from build123d import *

# Parameters (mm, degrees)
SKETCH1_W                  = 174
SKETCH1_H                  = 18
BOSS_EXTRUDE1_DEPTH        = 46
SKETCH3_W                  = 126
SKETCH3_H                  = 46
CUT_EXTRUDE1_DEPTH         = 4
SKETCH4_R                  = 7
BOSS_EXTRUDE2_DEPTH        = 14
SKETCH5_R                  = 14
SKETCH5_R_2                = 7
BOSS_EXTRUDE3_DEPTH        = 2
RIB1_REACH                 = 162.545
SKETCH6_WALL_W             = 359.980893116
SKETCH6_WALL_H             = 10
FILLET1_R                  = 2
FILLET2_R                  = 2
FILLET3_R                  = 2
F_10_0_10_DIAMETER_HOLE5_D = 10


with BuildPart() as part:
    # Sketch1 → Boss-Extrude1 (new body)
    with BuildSketch(Plane.XY):
        with Locations((54.12605042, 9)):
            Rectangle(SKETCH1_W, SKETCH1_H)
    extrude(amount=-BOSS_EXTRUDE1_DEPTH)

    # Sketch3 → Cut-Extrude1 (cut)
    with BuildSketch(Plane(origin=(0, 18, 0), x_dir=(1, 0, 0), z_dir=(0, 1, 0))):
        with Locations((54.12605042, 23)):
            Rectangle(SKETCH3_W, SKETCH3_H)
    extrude(amount=-CUT_EXTRUDE1_DEPTH, mode=Mode.SUBTRACT)

    # Sketch4 → Boss-Extrude2 (add)
    with BuildSketch(Plane(origin=(86.12605042, 0, 0), x_dir=(0, 0, -1), z_dir=(1, 0, 0))):
        with BuildLine():
            Line((46, 14), (0, 14))
            Line((0, 14), (0, 50))
            ThreePointArc((0, 50), (23, 73), (46, 50))
            Line((46, 50), (46, 14))
        make_face()
        with Locations((23, 50)):
            Circle(SKETCH4_R, mode=Mode.SUBTRACT)
    extrude(amount=-BOSS_EXTRUDE2_DEPTH)

    # Sketch5 → Boss-Extrude3 (add)
    with BuildSketch(Plane.ZY.offset(-72.12605042)):
        with Locations((-23, 50)):
            Circle(SKETCH5_R)
        with Locations(Location((-23, 50, 0), (0, 0, 180))):
            Circle(SKETCH5_R_2, mode=Mode.SUBTRACT)
    extrude(amount=BOSS_EXTRUDE3_DEPTH)

    # Sketch6 wall → Rib1 (add, up to next)
    with BuildSketch(Plane(origin=(101.62605042, 28, -23), x_dir=(-0.840296648224, 0.542126869822, 0), z_dir=(-0.542126869822, -0.840296648224, 0)), mode=Mode.PRIVATE) as rib1_sk1:
        Rectangle(SKETCH6_WALL_W, SKETCH6_WALL_H)
    rib1_tool1 = extrude(rib1_sk1.sketch, amount=RIB1_REACH, mode=Mode.PRIVATE) - part.part
    add(rib1_tool1.solids().sort_by_distance((101.62605042, 28, -23))[0])

    # Mirror4: part across plane


with BuildPart() as part_1:
    add(part.part)
    add(part.part.mirror(Plane(origin=(54.12605042, 0, 0), x_dir=(0, 0, 1), z_dir=(1, 0, 0))))

    # Fillet1
    fillet1_edges = [part_1.edges().sort_by_distance(p)[0] for p in [
        (-8.87394958, 14, -9),
        (22.12605042, 14, -37),
        (36.12605042, 14, -23),
        (22.12605042, 14, -9),
        (-8.87394958, 14, -37),
        (117.12605042, 14, -9),
        (72.12605042, 14, -23),
        (86.12605042, 14, -9),
        (86.12605042, 14, -37),
        (117.12605042, 14, -37),
    ]]
    fillet(fillet1_edges, radius=FILLET1_R)

    # Fillet2
    fillet2_edges = [part_1.edges().sort_by_distance(p)[0] for p in [
        (36.12605042, 50, -37),
    ]]
    fillet(fillet2_edges, radius=FILLET2_R - 0.0001)  # a hair under: the kernel refuses the full size

    # Fillet3
    fillet3_edges = [part_1.edges().sort_by_distance(p)[0] for p in [
        (72.12605042, 50, -37),
    ]]
    fillet(fillet3_edges, radius=FILLET3_R - 0.0001)  # a hair under: the kernel refuses the full size

    # Ø10.0 (10) Diameter Hole5 (through all)
    with Locations(Plane(origin=(0, 18, 0), x_dir=(1, 0, 0), z_dir=(0, 1, 0))):
        with Locations((-20.87394958, 35), (-20.87394958, 11), (129.12605042, 35), (129.12605042, 11)):
            Hole(F_10_0_10_DIAMETER_HOLE5_D / 2)


solid = part_1.part
Check sheet for the modelled part. Datum: model origin and axes. Units: mm. A direction names the side the tool comes from. Give positions to 0.01 mm unless a question says otherwise; leave off trailing zeros. Order: outer loops, then holes, each group sorted by start corner. A loop starts at its lowest first (then second) coordinate and runs counter-clockwise, first axis right, second up. Notation, with made-up numbers: (46, -27) - (58, -27) arc R8 cw to (58, -23) - close; hole circle Ø4 at (63.25, -20). An arc over 180 degrees is marked (long way). Answer as CSV lines item,"result".
1. Section check A-A (y = 11). Record the boundary of the cut face in (x, z).
Result sheet:
outline,"(-32.87, -46) - (141.13, -46) - (141.13, 0) - (-32.87, 0) - close; hole circle Ø10 at (-20.87, -35); hole circle Ø10 at (-20.87, -11); hole circle Ø10 at (129.13, -35); hole circle Ø10 at (129.13, -11)"
2. Mould release check, pull along X, two halves, no side actions. Record for faces 1 (the face through (-32.874, 9, -23)), 2 (the face through (72.126, 32, -23)), 3 (the face through (55, 9, -46)): released by +X, released by -X, zero draft, split by the parting line, or undercut.
Result sheet:
face 1,"released by -X"
face 2,"undercut"
face 3,"zero draft"
3. Section check C-C (y = 24.5). Record the boundary of the cut face in (x, z), then the cut area to 3 significant figures.
Result sheet:
outline,"(1.2, -28) - (22.13, -28) - (22.13, -46) - (36.13, -46) - (36.13, 0) - (22.13, 0) - (22.13, -18) - (1.2, -18) - close; (72.13, -46) - (86.13, -46) - (86.13, -28) - (107.05, -28) - (107.05, -18) - (86.13, -18) - (86.13, 0) - (72.13, 0) - close"
area,"1,710 mm²"
4. Go/stop test with flat-tipped pins: P1, Ø8, axis at x = 113, y = 18.5, coming from the +Z side; P2, Ø12, axis at x = 134, z = -16.5, coming from the +Y side; P3, Ø10, axis at y = 50, z = -26, coming from the -X side. Record where each tip stops, or that it passes through.
Result sheet:
P1,"z = -18"
P2,"y = 18"
P3,"x = 22.13"
5. Section check D-D (z = -11). State how many separate pieces and enclosed holes the cut face has, then the cut area to 3 significant figures.
Result sheet:
separate pieces,"3"
enclosed holes,"0"
area,"3,890 mm²"
6. Section check B-B (x = 24.5). Record the boundary of the cut face in (y, z).
Result sheet:
outline,"(0, -46) - (50, -46) arc R23 ccw to (50, 0) - (0, 0) - close; hole circle Ø14 at (50, -23)"
7. Scan lines: probe 1 along X at (y, z) = (12, -35); probe 2 along X at (y, z) = (26.5, -38.5); probe 3 along Y at (x, z) = (70.75, -23). Record each from-to range of solid material in increasing order. Write a range as from..to.
Result sheet:
probe 1,"-32.87..-25.87, -15.87..124.13, 134.13..141.13"
probe 2,"22.13..36.13, 72.13..86.13"
probe 3,"0..14.1, 35.9..43, 57..64.1"
8. Tool access check on faces 4 (the face through (36.126, 32, -23)), 5 (the face through (54, 14, -23)), 6 (the face through (101, 14, -37)), 7 (the face through (129, 18, -23)), 8 (the face through (98, 21, -18)). Record the directions out of +Z, -Z, +X, -X, +Y, -Y that give a thin tool (end or side, any length) a straight path to the whole face; none if there is none.
Result sheet:
face 4,"none"
face 5,"+Z, -Z, +Y"
face 6,"-Z, +Y"
face 7,"+Z, -Z, +X, +Y"
face 8,"+Z, +Y"
